from build123d import *

# Parameters (mm, degrees)
SKETCH_1_W          = 50
SKETCH_1_H          = 60
EXTRUDE_1_DEPTH     = 6
SKETCH_2_W          = 30
SKETCH_2_H          = 17
EXTRUDE_2_DEPTH     = 65
SKETCH_3_W          = 45
SKETCH_3_H          = 30
EXTRUDE_3_DEPTH     = 6
SKETCH_4_W          = 18
SKETCH_4_H          = 13
CUT_EXTRUDE_1_DEPTH = 10
SKETCH_5_W          = 24
SKETCH_5_H          = 5
CUT_EXTRUDE_2_DEPTH = 7
SKETCH_6_W          = 45
SKETCH_6_H          = 6
CUT_EXTRUDE_3_DEPTH = 6.5
SKETCH_7_W          = 45
SKETCH_7_H          = 6
CUT_EXTRUDE_4_DEPTH = 6.5


with BuildPart() as part:
    # Эскиз1 → Бобышка-Вытянуть1 (new body)
    with BuildSketch(Plane.XY):
        Rectangle(SKETCH_1_W, SKETCH_1_H)
    extrude(amount=EXTRUDE_1_DEPTH)

    # Эскиз2 → Бобышка-Вытянуть2 (add)
    with BuildSketch(Plane.XY.offset(6)):
        Rectangle(SKETCH_2_W, SKETCH_2_H)
    extrude(amount=EXTRUDE_2_DEPTH)

    # Эскиз3 → Бобышка-Вытянуть3 (add)
    with BuildSketch(Plane.XY.offset(71)):
        Rectangle(SKETCH_3_W, SKETCH_3_H)
    extrude(amount=EXTRUDE_3_DEPTH)

    # Эскиз4 → Вырез-Вытянуть1 (cut)
    with BuildSketch(Plane.ZY.offset(15)):
        with Locations((42, -2)):
            Rectangle(SKETCH_4_W, SKETCH_4_H)
    extrude(amount=-CUT_EXTRUDE_1_DEPTH, mode=Mode.SUBTRACT)

    # Эскиз5 → Вырез-Вытянуть2 (cut)
    with BuildSketch(Plane(origin=(15, 0, 0), x_dir=(0, 0, -1), z_dir=(1, 0, 0))):
        with Locations((-38, 6)):
            Rectangle(SKETCH_5_W, SKETCH_5_H)
    extrude(amount=-CUT_EXTRUDE_2_DEPTH, mode=Mode.SUBTRACT)

    # Эскиз6 → Вырез-Вытянуть3 (cut)
    with BuildSketch(Plane(origin=(0, 15, 0), x_dir=(1, 0, 0), z_dir=(0, 1, 0))):
        with Locations((0, -74)):
            Rectangle(SKETCH_6_W, SKETCH_6_H)
    extrude(amount=-CUT_EXTRUDE_3_DEPTH, mode=Mode.SUBTRACT)

    # Эскиз7 → Вырез-Вытянуть4 (cut)
    with BuildSketch(Plane.XZ.offset(15)):
        with Locations((0, 74)):
            Rectangle(SKETCH_7_W, SKETCH_7_H)
    extrude(amount=-CUT_EXTRUDE_4_DEPTH, mode=Mode.SUBTRACT)


solid = part.part
For this review, take the finished solid that the model builds, in its own axes (mm). A direction names the side the tool comes from. Coordinates: 2 decimals unless noted, no trailing zeros. Loops run counter-clockwise (first coordinate to the right, second up) from the corner with the lowest first, then second, coordinate; pieces in that order, holes last. Notation, with made-up numbers: (65.25, 38) -> (75.25, 38) arc R31 ccw to (75.25, 72) -> close; hole circle Ø6 at (-37, 32.25). An arc over 180 degrees is marked (long way). Write each question's results on one line, items separated by ' | '.
Q1. Add section C-C, the plane x = -11. State the section outline as (y, z) points.
Taken from the geometry:
outline: (-30, 0) -> (30, 0) -> (30, 6) -> (8.5, 6) -> (8.5, 77) -> (-8.5, 77) -> (-8.5, 51) -> (4.5, 51) -> (4.5, 33) -> (-8.5, 33) -> (-8.5, 6) -> (-30, 6) -> close
Q2. To check wall thickness, follow line 1 along Z through (x, y) = (-14, 2.5); line 2 along Z through (x, y) = (-3.5, -22.5); line 3 along Y through (x, z) = (-4.5, 53.5). State the ranges of each line that lie inside material, in increasing order. Write a range as [from, to].
Taken from the geometry:
line 1: [0, 33], [51, 77] | line 2: [0, 6] | line 3: [-8.5, 8.5]
Q3. For pin 1 Ø5 at (x, z) = (-15, 51) entering from +Y; pin 2 Ø1.8 at (y, z) = (-0.5, 72.5) entering from -X; pin 3 Ø3 at (y, z) = (-2, 74.5) entering from +X; pin 4 Ø8 at (x, y) = (4.5, -23.5) entering from -Z, all flat-tipped, find the tip position at first contact; note any pin that passes through.
Taken from the geometry:
pin 1: y = 8.5 | pin 2: x = -22.5 | pin 3: x = 22.5 | pin 4: z = 0
Q4. Add section D-D, the plane z = 41.5. State the section outline as (x, y) points, then the cut area to 3 significant figures.
Taken from the geometry:
outline: (-15, 4.5) -> (-5, 4.5) -> (-5, -8.5) -> (15, -8.5) -> (15, 3.5) -> (8, 3.5) -> (8, 8.5) -> (-15, 8.5) -> close | area: 345 mm²
Q5. Add section A-A, the plane x = -19.5. State the section outline as (y, z) points.
Taken from the geometry:
outline: (-30, 0) -> (30, 0) -> (30, 6) -> (-30, 6) -> close; (-8.5, 71) -> (8.5, 71) -> (8.5, 77) -> (-8.5, 77) -> close
Q6. Add section B-B, the plane y = -1. State the section outline as (x, z) points, then the cut area to 3 significant figures.
Taken from the geometry:
outline: (-25, 0) -> (25, 0) -> (25, 6) -> (15, 6) -> (15, 71) -> (22.5, 71) -> (22.5, 77) -> (-22.5, 77) -> (-22.5, 71) -> (-15, 71) -> (-15, 51) -> (-5, 51) -> (-5, 33) -> (-15, 33) -> (-15, 6) -> (-25, 6) -> close | area: 2,340 mm²
Q7. Machinability: for faces 5 (the flat face through (5, -8.5, 42)), 6 (the flat face through (-10, 4.5, 42)), 7 (the flat face through (0, 8.5, 41)), 8 (the flat face through (12, 3.5, 38)), which of the approach directions +Z, -Z, +X, -X, +Y, -Y give a long, thin tool a straight path to every point of the face, cutting with its end or side? Answer none if there is none.
Taken from the geometry:
face 5: +Z, +X, -X, -Y | face 6: -X, -Y | face 7: +Z, +X, -X, +Y | face 8: +X, +Y
Q8. Mouldability with a two-part tool opening along Z and no side actions: class faces 1 (the flat face through (-10, -2, 51)), 2 (the flat face through (12, 6, 26)), 3 (the flat face through (-25, 0, 3)), 4 (the flat face through (0, 0, 77)) as +Z half, -Z half, draft (parallel to the pull), parting line (faces both ways), or undercut.
Taken from the geometry:
face 1: undercut | face 2: undercut | face 3: draft | face 4: +Z half
